from build123d import *

# Parameters (mm, degrees)
F0_W     = 83.2
F0_H     = 13.6
F1_DEPTH = 33.5
F4_DEPTH = 69.2
F5_W     = 32.4
F5_H     = 3.6
F6_DEPTH = 8
F7_R     = 3.45
F7_W     = 14.6
F7_H     = 7.2
F8_DEPTH = 2.8


with BuildPart() as f1:
    # F0 (on Front) → F1 (new body)
    with BuildSketch(Plane.XZ):
        Rectangle(F0_W, F0_H)
    extrude(amount=F1_DEPTH)

    # F3 (on offset) → F4 (join)
    with BuildSketch(Plane(origin=(-34, 0, 0), x_dir=(0, -1, 0), z_dir=(-1, 0, 0))):
        Polygon((9.8, 10.4), (9.8, 6.8), (16.8, 6.8), (12.3, 10.4), align=None)
    extrude(amount=-F4_DEPTH)

    # F5 (on face) → F6 (cut, up to face)
    with BuildSketch(Plane(origin=(0, -9.8, 0), x_dir=(-1, 0, 0), z_dir=(0, 1, 0))):
        with Locations((-1.1, 8.6)):
            Rectangle(F5_W, F5_H)
    extrude(amount=-F6_DEPTH, mode=Mode.SUBTRACT)

    # F7 (on face) → F8 (join)
    with BuildSketch(Plane.XZ.offset(33.5)):
        with Locations((-28.95, -1.25)):
            Circle(F7_R)
        with Locations((-14.75, -1.25)):
            Circle(F7_R)
        with Locations((4.3, -1.25)):
            Rectangle(F7_W, F7_H)
        with Locations((26.8, -1.25)):
            Rectangle(F7_W, F7_H)
    extrude(amount=F8_DEPTH)


solid = f1.part
Check sheet for the modelled part. Datum: model origin and axes. Units: mm. A direction names the side the tool comes from. Give positions to 0.01 mm unless a question says otherwise; leave off trailing zeros. Write each loop counter-clockwise with the first axis right and the second up, starting at its lowest first coordinate (ties: lowest second). Pieces come first, ordered by that corner, then holes. Notation, with made-up numbers: (26, 55.5) -> (61, 55.5) arc R9 ccw to (61, 68.5) -> close; hole circle Ø11 at (-35.75, 87.25). An arc over 180 degrees is marked (long way). Use one line per item in the form item = value. Start each with the question number.
1. Section check A-A (z = -1.25). Record the cut outline in (x, y), and give its area (3 significant figures).
2. Section check D-D (z = 9.25). Record the cut outline in (x, y).
3. Access from +Z, -Z, +X, -X, +Y, -Y to the whole of each face (thin tool, end or side, straight path). Record for faces 5 (the flat face through (4, -35, 2.35)), 6 (the flat face through (27, -35, -4.85)), 7 (the flat face through (17.3, -12, 8)), 8 (the flat face through (35.2, -12, 8)), 9 (the flat face through (11.6, -35, -1)).
4. Thickness scan on line 1 along Y through (x, z) = (-36.5, -4.5); line 2 along Z through (x, y) = (2, -15). Record the ranges inside material, lowest first. Write a range as from..to.
5. Section check B-B (x = 29). Record the cut outline in (y, z).
6. Go/stop test with flat-tipped pins: P1, Ø1.1, axis at y = -14, z = 8.5, coming from the +X side; P2, Ø0.8, axis at y = -34.5, z = -2, coming from the +X side; P3, Ø5, axis at x = -9, y = -30.5, coming from the +Z side. Record where each tip stops, or that it passes through.
7. Mould release check, pull along X, two halves, no side actions. Record for faces 1 (the flat face through (-15.1, -12, 8)), 2 (the flat face through (34.1, -35, -1)), 3 (the flat face through (-15, -36.3, -1)), 4 (the flat face through (19.5, -35, -1)): pulls with the +X half, pulls with the -X half, needs draft (parallel to the pull), parting line crosses it, or undercut.
8. Section check C-C (y = -14). Record the cut outline in (x, z), and give its area (3 significant figures).
Conclusion:
q1.outline = (-41.6, -33.5) -> (-32.4, -33.5) -> (-32.4, -36.3) -> (-25.5, -36.3) -> (-25.5, -33.5) -> (-18.2, -33.5) -> (-18.2, -36.3) -> (-11.3, -36.3) -> (-11.3, -33.5) -> (-3, -33.5) -> (-3, -36.3) -> (11.6, -36.3) -> (11.6, -33.5) -> (19.5, -33.5) -> (19.5, -36.3) -> (34.1, -36.3) -> (34.1, -33.5) -> (41.6, -33.5) -> (41.6, 0) -> (-41.6, 0) -> close
q1.area = 2,910 mm²
q2.outline = (-34, -13.74) -> (-15.1, -13.74) -> (-15.1, -9.8) -> (-34, -9.8) -> close; (17.3, -13.74) -> (35.2, -13.74) -> (35.2, -9.8) -> (17.3, -9.8) -> close
q3.face_5 = +Z, +X, -X, -Y
q3.face_6 = -Z, +X, -X, -Y
q3.face_7 = +Z, +Y, -Y
q3.face_8 = +Z, +X, +Y, -Y
q3.face_9 = +Z, -Z, -Y
q4.line_1 = -33.5..0
q4.line_2 = -6.8..6.8
q5.outline = (-36.3, -4.85) -> (-33.5, -4.85) -> (-33.5, -6.8) -> (0, -6.8) -> (0, 6.8) -> (-9.8, 6.8) -> (-9.8, 10.4) -> (-12.3, 10.4) -> (-16.8, 6.8) -> (-33.5, 6.8) -> (-33.5, 2.35) -> (-36.3, 2.35) -> close
q6.P1 = 35.2
q6.P2 = 34.1
q6.P3 = 6.8
q7.face_1 = undercut
q7.face_2 = pulls with the +X half
q7.face_3 = needs draft
q7.face_4 = undercut
q8.outline = (-41.6, -6.8) -> (41.6, -6.8) -> (41.6, 6.8) -> (35.2, 6.8) -> (35.2, 9.04) -> (17.3, 9.04) -> (17.3, 6.8) -> (-15.1, 6.8) -> (-15.1, 9.04) -> (-34, 9.04) -> (-34, 6.8) -> (-41.6, 6.8) -> close
q8.area = 1,210 mm²
